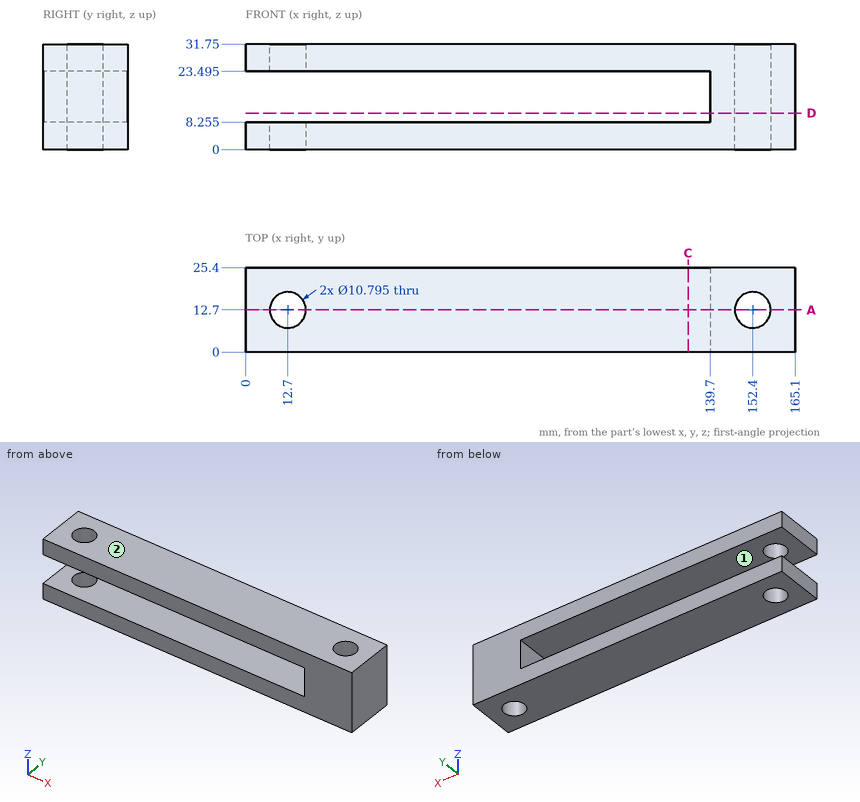
Can you work these out from the drawing? Everything is in mm from the part's minimum corner. A direction names the side the tool comes from. Coordinates: 2 decimals unless noted, no trailing zeros. Write each loop counter-clockwise with the first axis right and the second up, starting at its lowest first coordinate (ties: lowest second). Pieces come first, ordered by that corner, then holes. Notation, with made-up numbers: (-26, 71.25) -> (28, 71.25) arc R13 cw to (28, 77.25) -> close; hole circle Ø3 at (-10.75, 49). An arc over 180 degrees is marked (long way). Write each question's results on one line, items separated by ' | '. Start each with the question number.
Q1. If I drill on probe 1 along X at (y, z) = (13, 7); probe 2 along Z at (x, y) = (40, 20.25) (3 decimals); probe 3 along X at (y, z) = (14, 27), over which ranges is the centre line in solid material (lowest first)?
Q2. I'm going to push flat-ended pins straight in: pin 1 (1 mm diameter, centred on x = 119.5, z = 21.5, fed in from -Y); pin 2 (3 mm diameter, centred on y = 17.5, z = 18, fed in from -X). Where does each tip first touch, or does it pass through?
Q3. Imagine slicing it at D-D (z = 11). Write out the boundary of the cut face in (x, y) (1 decimal).
Q4. On a 3-axis mill with a long thin cutter (end or side, diameter ignored), from which of +Z, -Z, +X, -X, +Y, -Y can I reach the whole of each face in a straight line? I mean the marked faces 1 and 2. Say none if no direction works.
Q5. Imagine slicing it at A-A (y = 12.7). State how many separate pieces and enclosed holes the cut face has, then the cut area to 3 significant figures.
Q6. Imagine slicing it at C-C (x = 133). Write out the boundary of the cut face in (y, z) (3 decimals).
Taken from the geometry:
1) probe 1: x = 0 to 7.31, 18.09 to 147.01, 157.79 to 165.1 | probe 2: z = 0 to 8.255, 23.495 to 31.75 | probe 3: x = 0 to 7.46, 17.94 to 147.16, 157.64 to 165.1
2) pin 1: passes through | pin 2: stops at x = 139.7
3) outline: (139.7, 0) -> (165.1, 0) -> (165.1, 25.4) -> (139.7, 25.4) -> close; hole circle Ø10.8 at (152.4, 12.7)
4) face 1: -X, +Y, -Y | face 2: +Z, +X, -X, +Y, -Y
5) separate pieces: 4 | enclosed holes: 0 | area: 2,590 mm^2
6) outline: (0, 0) -> (25.4, 0) -> (25.4, 8.255) -> (0, 8.255) -> close; (0, 23.495) -> (25.4, 23.495) -> (25.4, 31.75) -> (0, 31.75) -> close
